```python
from build123d import *

# Parameters (mm, degrees)
SKETCH1_W               = 101.6
SKETCH1_H               = 38.1
BOSS_EXTRUDE1_DEPTH     = 40
SKETCH2_W               = 16.891
SKETCH2_H               = 38.1
BOSS_EXTRUDE2_DEPTH     = 45
FILLET1_R               = 7.62
CUT_EXTRUDE1_DEPTH      = 134.829976089
CUT_EXTRUDE1_DEPTH_BACK = 134.829976089
CUT_EXTRUDE2_DEPTH      = 134.829976089
CUT_EXTRUDE2_DEPTH_BACK = 134.829976089
FILLET2_R               = 1.27
BOSS_EXTRUDE3_DEPTH     = 105
FILLET3_R               = 7.62
SKETCH9_W               = 101.6
SKETCH9_H               = 85
BOSS_EXTRUDE4_DEPTH     = 7.62
FILLET4_R               = 2.54


with BuildPart() as part:
    # Sketch1 → Boss-Extrude1 (new body)
    with BuildSketch(Plane(origin=(0, 0, 0), x_dir=(1, 0, 0), z_dir=(0, 1, 0))):
        Rectangle(SKETCH1_W, SKETCH1_H)
    extrude(amount=BOSS_EXTRUDE1_DEPTH)

    # Sketch2 → Boss-Extrude2 (add)
    with BuildSketch(Plane(origin=(0, 40, 0), x_dir=(1, 0, 0), z_dir=(0, 1, 0))):
        with Locations((-42.3545, 0)):
            Rectangle(SKETCH2_W, SKETCH2_H)
        with Locations((42.3545, 0)):
            Rectangle(SKETCH2_W, SKETCH2_H)
    extrude(amount=BOSS_EXTRUDE2_DEPTH)

    # Fillet1
    fillet1_edges = [part.edges().sort_by_distance(p)[0] for p in [
        (-33.909, 40, 0),
        (33.909, 40, 0),
    ]]
    fillet(fillet1_edges, radius=FILLET1_R)

    # Sketch6 → Cut-Extrude1 (cut, two sides: drawn at the far end of the back side and taken through both)
    with BuildSketch(Plane.ZY.offset(50.8).offset(-CUT_EXTRUDE1_DEPTH_BACK)):
        Polygon((-11.938, 0), (-11.938, 1.524), (-15.24, 1.524), (-15.24, 2.54), (-12.186712919, 5.593287081), (-7.360712919, 5.593287081), (-4.307425838, 2.54), (-4.307425838, 1.524), (-7.609425838, 1.524), (-7.609425838, 0), align=None)
    extrude(amount=CUT_EXTRUDE1_DEPTH + CUT_EXTRUDE1_DEPTH_BACK, mode=Mode.SUBTRACT)

    # Sketch5 → Cut-Extrude2 (cut, two sides: drawn at the far end of the back side and taken through both)
    with BuildSketch(Plane.ZY.offset(50.8).offset(-CUT_EXTRUDE2_DEPTH_BACK)):
        Polygon((7.863425838, 0), (7.863425838, 1.524), (4.561425838, 1.524), (4.561425838, 2.54), (7.614712919, 5.593287081), (12.440712919, 5.593287081), (15.494, 2.54), (15.494, 1.524), (12.192, 1.524), (12.192, 0), align=None)
    extrude(amount=CUT_EXTRUDE2_DEPTH + CUT_EXTRUDE2_DEPTH_BACK, mode=Mode.SUBTRACT)

    # Fillet2
    # the kernel refuses this fillet: 1.27 mm, written as the material it adds along each edge
    with BuildSketch(Plane(origin=(-50.8, 1.524, -15.24), x_dir=(0, 0, 1), z_dir=(1, 0, 0)), Plane(origin=(-50.8, 1.524, 4.561425838), x_dir=(0, 0, 1), z_dir=(1, 0, 0))) as fillet2_piece_1:
        with BuildLine():
            CenterArc((1.244340789, -1.27), FILLET2_R, 90, 78.463040967)
            Line((0, -1.016), (-0.024886816, -1.01092))
            ThreePointArc((-0.024886816, -1.01092), (-0.0254, -0.508), (-0.0254, 0))
            Line((-0.0254, 0), (0, 0.0254))
            Line((0, 0.0254), (1.244340789, 0.0254))
            Line((1.244340789, 0.0254), (1.244340789, 0))
        make_face()
    extrude(amount=101.6)
    with BuildSketch(Plane(origin=(-50.8, 1.524, -4.307425838), x_dir=(0, 1.0, -1.5744186357080854e-12), z_dir=(1, 0, 0)), Plane(origin=(-50.8, 1.524, 15.494), x_dir=(0, 1.0, -1.561305765338501e-12), z_dir=(1, 0, 0))) as fillet2_piece_2:
        with BuildLine():
            CenterArc((1.27, -1.244340789), FILLET2_R, 101.536959033, 78.463040967)
            Line((0, -1.244340789), (-0.0254, -1.244340789))
            Line((-0.0254, -1.244340789), (-0.0254, 0))
            Line((-0.0254, 0), (0, 0.0254))
            ThreePointArc((0, 0.0254), (0.508, 0.0254), (1.01092, 0.024886816))
            Line((1.01092, 0.024886816), (1.016, 0))
        make_face()
    extrude(amount=101.6)

    # Sketch8 → Boss-Extrude3 (add)
    with BuildSketch(Plane(origin=(0, 0, -19.05), x_dir=(-1, 0, 0), z_dir=(0, 0, -1))):
        Polygon((-33.909, 39.760810351), (-50.8, 39.760810351), (-50.8, 0), (50.8, 0), (50.8, 39.760810351), (33.909, 39.760810351), align=None)
        Polygon((-50.8, 85), (-50.8, 39.760810351), (-33.909, 39.760810351), (-33.909, 47.62), (-33.909, 85), align=None)
        Polygon((33.909, 47.62), (33.909, 39.760810351), (50.8, 39.760810351), (50.8, 85), (33.909, 85), align=None)
    extrude(amount=BOSS_EXTRUDE3_DEPTH)

    # Fillet3
    fillet3_edges = [part.edges().sort_by_distance(p)[0] for p in [
        (-33.909, 39.760810351, -71.55),
        (33.909, 39.760810351, -71.55),
    ]]
    fillet(fillet3_edges, radius=FILLET3_R)

    # Sketch9 → Boss-Extrude4 (add)
    with BuildSketch(Plane(origin=(0, 0, -124.05), x_dir=(-1, 0, 0), z_dir=(0, 0, -1))):
        with Locations((0, 42.5)):
            Rectangle(SKETCH9_W, SKETCH9_H)
    extrude(amount=BOSS_EXTRUDE4_DEPTH)

    # Fillet4
    fillet4_edges = [part.edges().sort_by_distance(p)[0] for p in [
        (33.909, 66.190405175, -124.05),
        (-33.909, 66.190405175, -124.05),
        (0, 39.760810351, -124.05),
        (-31.677153673, 41.992656678, -124.05),
        (31.677153673, 41.992656678, -124.05),
    ]]
    fillet(fillet4_edges, radius=FILLET4_R)


solid = part.part
```
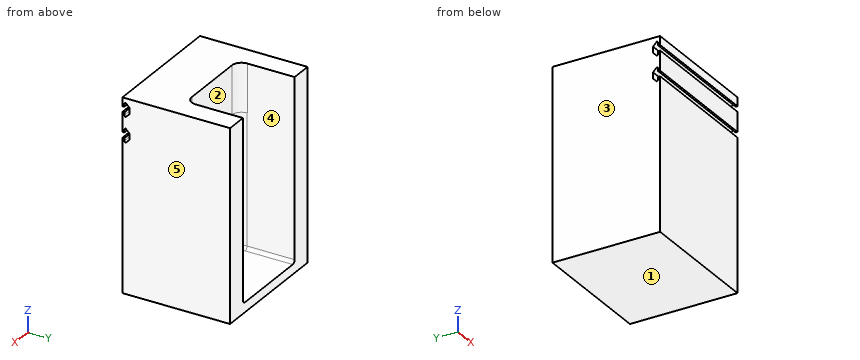
Work out the finished part from the listing and answer in its coordinate system (mm). Face numbers are marked on the shaded views. A direction names the side the tool comes from. Coordinates: 2 decimals unless noted, no trailing zeros. Write each loop counter-clockwise with the first axis right and the second up, starting at its lowest first coordinate (ties: lowest second). Pieces come first, ordered by that corner, then holes.
Q1. A cutting plane is placed at C-C, the plane y = 62. Give the vertices of the cut face in (x, z).
Q2. Which of the six approach directions +Z, -Z, +X, -X, +Y, -Y give full straight-line access (tool end or side, diameter ignored) to the marked faces 4 and 5?
Q3. Determine the mould class of the marked faces 1, 2 and 3 for opening direction X: released by +X, released by -X, zero draft, split by the parting line, or undercut.
Q4. Each of these flat-tipped pins is pushed along its axis until it touches: pin 1 Ø1 at (x, z) = (-26, -59) entering from +Y; pin 2 Ø2.5 at (x, z) = (10, -6.5) entering from +Y; pin 3 Ø13 at (x, y) = (14, 55) entering from +Z. Where does it stop, or does it pass through?
Q5. A cutting plane is placed at A-A, the plane z = -50. Give the vertices of the cut face in (x, y), then the cut area to 3 significant figures.
Q6. Find the intervals of material crossed by line 1 (X direction, y = 68, z = -21); line 2 (Z direction, x = -0.5, y = 5.5); line 3 (Z direction, x = -18.5, y = 75), in increasing order.
Findings below:
1. outline: (-50.8, -131.67) - (50.8, -131.67) - (50.8, 19.05) - (33.91, 19.05) - (33.91, -121.51) arc R2.54 cw to (31.37, -124.05) - (-31.37, -124.05) arc R2.54 cw to (-33.91, -121.51) - (-33.91, 19.05) - (-50.8, 19.05) - close
2. face 4: +Z, +Y
2. face 5: +Z, -Z, +X, +Y, -Y
3. face 1: zero draft
3. face 2: undercut
3. face 3: released by -X
4. pin 1: stops at y = 39.76
4. pin 2: stops at y = 40
4. pin 3: stops at z = -124.05
5. outline: (-50.8, 0) - (50.8, 0) - (50.8, 85) - (33.91, 85) - (33.91, 47.38) arc R7.62 cw to (26.29, 39.76) - (-26.29, 39.76) arc R7.62 cw to (-33.91, 47.38) - (-33.91, 85) - (-50.8, 85) - close
5. area: 5,590 mm2
6. line 1: x = -50.8 to -33.91, 33.91 to 50.8
6. line 2: z = -131.67 to -12.28, -7.27 to 7.52, 12.53 to 19.05
6. line 3: z = -131.67 to -124.05
